Work out the finished part from the listing and answer in its coordinate system (mm). A direction names the side the tool comes from. Give positions to 0.01 mm unless a question says otherwise; leave off trailing zeros. Write each loop counter-clockwise with the first axis right and the second up, starting at its lowest first coordinate (ties: lowest second). Pieces come first, ordered by that corner, then holes.
1) Find section C-C (x = 62). Determine the outline of the cut face in (y, z) (3 decimals), plus the area to 3 significant figures.
2) Find section B-B (x = 26.5). Determine the outline of the cut face in (y, z) (3 decimals).
3) Straight lines are drawn through the part: probe 1 along Z at (x, y) = (-37, 6) (3 decimals); probe 2 along Z at (x, y) = (61, 2.75) (3 decimals); probe 3 along X at (y, z) = (1, 16). For each, find the intervals that lie inside material, in ascending order.
4) Determine the mould class of faces 1 (the face through (61, 7, -21)), 2 (the face through (-12, 5, 21.375)), 3 (the face through (-79.271, 4.339, 14.535)) for opening direction Y: pulls with the +Y half, pulls with the -Y half, needs draft (parallel to the pull), parting line crosses it, or undercut.
5) Find section A-A (x = -48). Determine the outline of the cut face in (y, z) (3 decimals), plus the area to 4 significant figures.
6) A tool of negligible diameter and unlimited length cuts with its end or side. For faces 4 (the face through (-61.4, 5, 1)), 5 (the face through (17, 0, -21)), 6 (the face through (-77.57, 2.71, -20.92)), from which of +Z, -Z, +X, -X, +Y, -Y can it reach the whole face along a straight path? Write none if from no direction.
7) Given pin 1 Ø1.2 at (x, z) = (-15, -26.5) entering from -Y; pin 2 Ø5.5 at (x, z) = (58.5, -5) entering from -Y; pin 3 Ø1.5 at (x, z) = (79.5, -21) entering from -Y, each flat-ended and moving along its own axis, determine where each tip first touches the part or whether it passes through.
```python
from build123d import *

# Parameters (mm, degrees)
SKETCH2_W                 = 150
SKETCH2_H                 = 62.75
BOSS_EXTRUDE1_DEPTH       = 10
SKETCH3_W                 = 99.5
SKETCH3_H                 = 41
CUT_EXTRUDE1_DEPTH        = 11
SKETCH7_W                 = 70
SKETCH7_H                 = 4
CUT_EXTRUDE4_DEPTH        = 7
SKETCH8_R                 = 4
CUT_EXTRUDE5_DEPTH        = 11
SKETCH9_R                 = 6.5
CUT_EXTRUDE6_DEPTH        = 7
SKETCH10_R                = 3.5
CUT_EXTRUDE7_DEPTH        = 7
SKETCH11_W                = 8
SKETCH11_H                = 62.75
BOSS_EXTRUDE2_DEPTH       = 10
M3X0_5_TAPPED_HOLE2_D     = 2.5
M3X0_5_TAPPED_HOLE2_DEPTH = 25
M3X0_5_TAPPED_HOLE2_TIP   = 0.751075774
M3X0_5_TAPPED_HOLE3_D     = 2.5
M3X0_5_TAPPED_HOLE3_DEPTH = 21
M3X0_5_TAPPED_HOLE3_TIP   = 0.751075774
SKETCH28_R                = 1.5
CUT_EXTRUDE8_DEPTH        = 5.5
SKETCH29_R                = 8.814479729
CUT_EXTRUDE9_DEPTH        = 5


with BuildPart() as part:
    # Sketch2 → Boss-Extrude1 (new body)
    with BuildSketch(Plane(origin=(0, 0, 0), x_dir=(1, 0, 0), z_dir=(0, 1, 0))):
        Rectangle(SKETCH2_W, SKETCH2_H)
    extrude(amount=BOSS_EXTRUDE1_DEPTH)

    # Sketch3 → Cut-Extrude1 (cut, through all)
    with BuildSketch(Plane(origin=(0, 10, 0), x_dir=(1, 0, 0), z_dir=(0, 1, 0))):
        with Locations((-11.65, -0.875)):
            Rectangle(SKETCH3_W, SKETCH3_H)
    extrude(amount=-CUT_EXTRUDE1_DEPTH, mode=Mode.SUBTRACT)

    # Sketch7 → Cut-Extrude4 (cut)
    with BuildSketch(Plane.XZ):
        with Locations((-26.4, -26.575)):
            Rectangle(SKETCH7_W, SKETCH7_H)
    extrude(amount=-CUT_EXTRUDE4_DEPTH, mode=Mode.SUBTRACT)

    # Sketch8 → Cut-Extrude5 (cut, through all)
    with BuildSketch(Plane(origin=(0, 10, 0), x_dir=(1, 0, 0), z_dir=(0, 1, 0))):
        with Locations((62.5, 1.625)):
            Circle(SKETCH8_R)
    extrude(amount=-CUT_EXTRUDE5_DEPTH, mode=Mode.SUBTRACT)

    # Sketch9 → Cut-Extrude6 (cut)
    with BuildSketch(Plane.XZ):
        with Locations((61, -20.625)):
            Circle(SKETCH9_R)
    extrude(amount=-CUT_EXTRUDE6_DEPTH, mode=Mode.SUBTRACT)

    # Sketch10 → Cut-Extrude7 (cut)
    with BuildSketch(Plane(origin=(0, 0, 0), x_dir=(-1, 0, 0), z_dir=(0, -1, 0))):
        with Locations((-62, -14.625)):
            Circle(SKETCH10_R)
    extrude(amount=-CUT_EXTRUDE7_DEPTH, mode=Mode.SUBTRACT)

    # Sketch11 → Boss-Extrude2 (add, through all)
    with BuildSketch(Plane(origin=(0, 10, 0), x_dir=(1, 0, 0), z_dir=(0, 1, 0))):
        with Locations((-79, 0)):
            Rectangle(SKETCH11_W, SKETCH11_H)
        with Locations((79, 0)):
            Rectangle(SKETCH11_W, SKETCH11_H)
    extrude(amount=-BOSS_EXTRUDE2_DEPTH)

    # M3x0.5 Tapped Hole2
    with Locations(Plane(origin=(0, -15.6875, 15.6875), x_dir=(1, 0, 0), z_dir=(0, -0.707106781, 0.707106781))):
        with Locations((79, 6.12547526)):
            Hole(M3X0_5_TAPPED_HOLE2_D / 2, depth=M3X0_5_TAPPED_HOLE2_DEPTH)
            with Locations((0, 0, -(M3X0_5_TAPPED_HOLE2_DEPTH + M3X0_5_TAPPED_HOLE2_TIP / 2))):  # 118° drill point
                Cone(0, M3X0_5_TAPPED_HOLE2_D / 2, M3X0_5_TAPPED_HOLE2_TIP, mode=Mode.SUBTRACT)

    # M3x0.5 Tapped Hole3
    with Locations(Plane(origin=(0, -15.6875, 15.6875), x_dir=(-1, 0, 0), z_dir=(0, -0.707106781, 0.707106781))):
        with Locations((79, -12.12547526)):
            Hole(M3X0_5_TAPPED_HOLE3_D / 2, depth=M3X0_5_TAPPED_HOLE3_DEPTH)
            with Locations((0, 0, -(M3X0_5_TAPPED_HOLE3_DEPTH + M3X0_5_TAPPED_HOLE3_TIP / 2))):  # 118° drill point
                Cone(0, M3X0_5_TAPPED_HOLE3_D / 2, M3X0_5_TAPPED_HOLE3_TIP, mode=Mode.SUBTRACT)

    # Sketch28 → Cut-Extrude8 (cut)
    with BuildSketch(Plane.XZ):
        with Locations((79, -21.375)):
            Circle(SKETCH28_R)
        with Locations((-79, -21.375)):
            Circle(SKETCH28_R)
    extrude(amount=-CUT_EXTRUDE8_DEPTH, mode=Mode.SUBTRACT)

    # Sketch29 → Cut-Extrude9 (cut)
    with BuildSketch(Plane.XZ):
        with Locations((62.5, -1.625)):
            Circle(SKETCH29_R)
    extrude(amount=-CUT_EXTRUDE9_DEPTH, mode=Mode.SUBTRACT)


solid = part.part
```
Results:
1. outline: (0, -31.375) - (10, -31.375) - (10, -5.594) - (5, -5.594) - (5, -10.425) - (0, -10.425) - (0, -14.202) - (7, -14.202) - (7, -27.048) - (0, -27.048) - close; (0, 7.175) - (5, 7.175) - (5, 2.344) - (10, 2.344) - (10, 31.375) - (0, 31.375) - (0, 18.125) - (7, 18.125) - (7, 11.125) - (0, 11.125) - close
1. area: 361 mm2
2. outline: (0, -31.375) - (10, -31.375) - (10, -19.625) - (0, -19.625) - close; (0, 21.375) - (10, 21.375) - (10, 31.375) - (0, 31.375) - close
3. probe 1: z = -31.375 to -28.575, -24.575 to -19.625, 21.375 to 31.375
3. probe 2: z = -31.375 to -27.125, -14.125 to -10.311, 7.061 to 11.271, 17.979 to 31.375
3. probe 3: x = -83 to -80.25, -77.75 to -61.4, 38.1 to 58.78, 65.22 to 83
4. face 1: pulls with the -Y half
4. face 2: needs draft
4. face 3: undercut
5. outline: (0, -31.375) - (10, -31.375) - (10, -19.625) - (0, -19.625) - (0, -24.575) - (7, -24.575) - (7, -28.575) - (0, -28.575) - close; (0, 21.375) - (10, 21.375) - (10, 31.375) - (0, 31.375) - close
5. area: 189.5 mm2
6. face 4: +Y, -Y
6. face 5: +Z, -Z, +X, -X, -Y
6. face 6: -Y
7. pin 1: stops at y = 7
7. pin 2: stops at y = 5
7. pin 3: stops at y = 5.5
